Design review of the part built by this model. Coordinates are the model's own, in mm. Give positions to 0.01 mm unless a question says otherwise; leave off trailing zeros. Write each loop counter-clockwise with the first axis right and the second up, starting at its lowest first coordinate (ties: lowest second). Pieces come first, ordered by that corner, then holes.
```python
from build123d import *

# Parameters (mm, degrees)
SKETCH1_W           = 20
SKETCH1_H           = 20
BOSS_EXTRUDE1_DEPTH = 100
FILLET1_R           = 3
SKETCH4_R           = 2
CUT_EXTRUDE1_DEPTH  = 10


with BuildPart() as part:
    # Sketch1 → Boss-Extrude1 (new body)
    with BuildSketch(Plane(origin=(0, 0, 0), x_dir=(1, 0, 0), z_dir=(0, 1, 0))):
        Rectangle(SKETCH1_W, SKETCH1_H)
    extrude(amount=BOSS_EXTRUDE1_DEPTH)

    # Fillet1
    fillet1_edges = [part.edges().sort_by_distance(p)[0] for p in [
        (-10, 50, -10),
        (10, 50, -10),
        (10, 50, 10),
        (-10, 50, 10),
    ]]
    fillet(fillet1_edges, radius=FILLET1_R)

    # Sketch4 → Cut-Extrude1 (cut)
    with BuildSketch(Plane(origin=(0, 100, 0), x_dir=(1, 0, 0), z_dir=(0, 1, 0))):
        with Locations(Location((0, 0, 0), (0, 0, 270))):
            Circle(SKETCH4_R)
    cut_extrude1 = extrude(amount=-CUT_EXTRUDE1_DEPTH, mode=Mode.SUBTRACT)

    # Mirror1: Cut-Extrude1 across plane
    add(cut_extrude1.mirror(Plane.ZX.offset(50)), mode=Mode.SUBTRACT)


solid = part.part
```
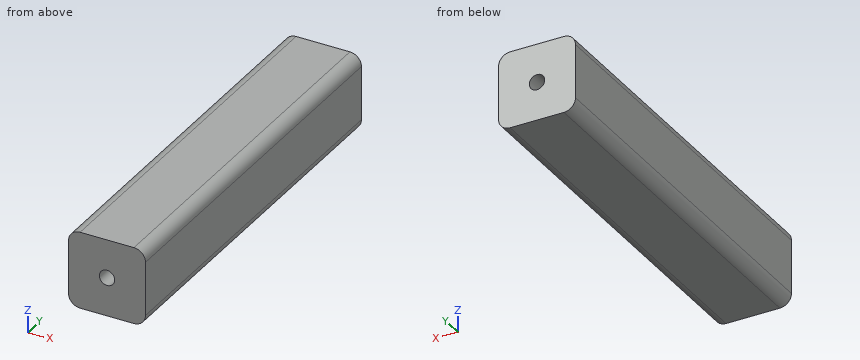
(1) Clearance check with flat-ended pins moving along their axes: P1, Ø1.2, axis at x = 0, z = -1, coming from the +Y side; P2, Ø5, axis at x = 0, z = 0, coming from the -Y side; P3, Ø3, axis at x = 0, z = 0, coming from the -Y side. State where each tip first meets the part, or that it passes through.
Resolved:
P1: stops at y = 90
P2: stops at y = 0
P3: stops at y = 10
(2) To check wall thickness, follow L1, parallel to X at y = 2.5, z = 0; L2, parallel to Y at x = -1, z = 0; L3, parallel to Z at x = -1.5, y = 7. State the ranges of each line that lie inside material, in increasing order.
Resolved:
L1: x = -10 to -2, 2 to 10
L2: y = 10 to 90
L3: z = -10 to -1.32, 1.32 to 10
(3) Consider section D-D, the plane z = -8. Give the boundary of the cut face in (x, y), then the cut area to 3 significant figures.
Resolved:
outline: (-9.83, 0) - (9.83, 0) - (9.83, 100) - (-9.83, 100) - close
area: 1,970 mm2
(4) Consider section A-A, the plane z = 0. Give the boundary of the cut face in (x, y).
Resolved:
outline: (-10, 0) - (-2, 0) - (-2, 10) - (2, 10) - (2, 0) - (10, 0) - (10, 100) - (2, 100) - (2, 90) - (-2, 90) - (-2, 100) - (-10, 100) - close
(5) Consider section C-C, the plane y = 83.5. Give the boundary of the cut face in (x, z), then the cut area to 3 significant figures.
Resolved:
outline: (-10, -7) arc R3 ccw to (-7, -10) - (7, -10) arc R3 ccw to (10, -7) - (10, 7) arc R3 ccw to (7, 10) - (-7, 10) arc R3 ccw to (-10, 7) - close
area: 392 mm2
(6) Consider section B-B, the plane x = 0. Give the boundary of the cut face in (y, z), then the cut area to 3 significant figures.
Resolved:
outline: (0, -10) - (100, -10) - (100, -2) - (90, -2) - (90, 2) - (100, 2) - (100, 10) - (0, 10) - (0, 2) - (10, 2) - (10, -2) - (0, -2) - close
area: 1,920 mm2
